Geometry: final body of the model. Coordinates: model frame, mm. Face numbers are marked on the shaded views. A direction names the side the tool comes from. Coordinates: 2 decimals unless noted, no trailing zeros. Loops run counter-clockwise (first coordinate to the right, second up) from the corner with the lowest first, then second, coordinate; pieces in that order, holes last. Notation, with made-up numbers: (28, 9.25) - (53, 9.25) arc R20 cw to (53, 45.25) - close; hole circle Ø5 at (47.5, -16.5). An arc over 180 degrees is marked (long way). Answer in a Markdown table with one row per item.
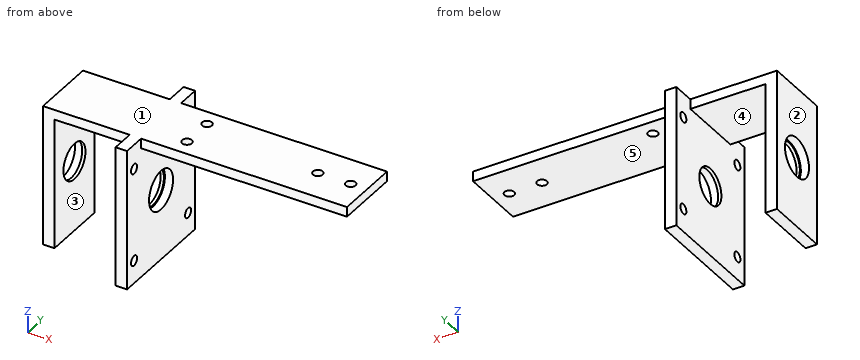
from build123d import *

# Parameters (mm, degrees)
SKETCH_1_W          = 20
SKETCH_1_H          = 20
SKETCH_1_R          = 1.5
SKETCH_1_W_2        = 23
SKETCH_1_W_3        = 3.5
EXTRUDE_1_DEPTH     = 3
EXTRUDE_2_DEPTH     = 40
SKETCH_2_R          = 1.5
CUT_EXTRUDE_1_DEPTH = 10
SKETCH_1_4_W        = 3.5
SKETCH_1_4_H        = 20
EXTRUDE_3_DEPTH     = 40
SKETCH_3_R          = 6
CUT_EXTRUDE_2_DEPTH = 38
SKETCH_4_R          = 6
SKETCH_4_R_2        = 5.5
EXTRUDE_4_DEPTH     = 1
SKETCH_5_R          = 6
SKETCH_5_R_2        = 5.5
EXTRUDE_5_DEPTH     = 1
SKETCH_7_R          = 1.5
CUT_EXTRUDE_4_DEPTH = 5


with BuildPart() as part:
    # Sketch 1 → Extrude 1 (new body)
    with BuildSketch(Plane.XY):
        Polygon((-10, -10.145751311), (-10, 9.854248689), (-53, 9.854248689), (-53, -0.145751311), (-53, -10.145751311), align=None)
        with Locations((0, -0.145751311)):
            Rectangle(SKETCH_1_W, SKETCH_1_H)
        with Locations((-5, -0.145751311)):
            Circle(SKETCH_1_R, mode=Mode.SUBTRACT)
        with Locations((5, -0.145751311)):
            Circle(SKETCH_1_R, mode=Mode.SUBTRACT)
        Polygon((-53, -0.145751311), (-53, 9.854248689), (-53, 16.854248689), (-56.5, 16.854248689), (-56.5, 9.854248689), (-56.5, -10.145751311), (-56.5, -17.145751311), (-53, -17.145751311), (-53, -10.145751311), align=None)
        with Locations((-68, -0.145751311)):
            Rectangle(SKETCH_1_W_2, SKETCH_1_H)
        with Locations((-81.25, -0.145751311)):
            Rectangle(SKETCH_1_W_3, SKETCH_1_H)
    extrude(amount=EXTRUDE_1_DEPTH)

    # Sketch 1_3 → Extrude 2 (add)
    with BuildSketch(Plane.XY):
        Polygon((-56.5, 16.854248689), (-56.5, 9.854248689), (-56.5, -10.145751311), (-56.5, -17.145751311), (-53, -17.145751311), (-53, -0.145751311), (-53, 16.854248689), align=None)
    extrude(amount=-EXTRUDE_2_DEPTH)

    # Sketch 2 → Cut-Extrude 1 (cut, symmetric)
    with BuildSketch(Plane(origin=(-53, 0, 0), x_dir=(0, 0, -1), z_dir=(-1, 0, 0))):
        with Locations((33, -13.354248689)):
            Circle(SKETCH_2_R)
        with Locations((4.5, 13.645751311)):
            Circle(SKETCH_2_R)
        with Locations((33, 13.645751311)):
            Circle(SKETCH_2_R)
        with Locations((4.5, -13.354248689)):
            Circle(SKETCH_2_R)
    extrude(amount=CUT_EXTRUDE_1_DEPTH, both=True, mode=Mode.SUBTRACT)

    # Sketch 1_4 → Extrude 3 (add)
    with BuildSketch(Plane.XY):
        with Locations((-81.25, -0.145751311)):
            Rectangle(SKETCH_1_4_W, SKETCH_1_4_H)
    extrude(amount=-EXTRUDE_3_DEPTH)

    # Sketch 3 → Cut-Extrude 2 (cut)
    with BuildSketch(Plane.ZY.offset(83)):
        with Locations((-18.5, -0.145751311)):
            Circle(SKETCH_3_R)
    extrude(amount=-CUT_EXTRUDE_2_DEPTH, mode=Mode.SUBTRACT)

    # Sketch 4 → Extrude 4 (add)
    with BuildSketch(Plane.ZY.offset(56.5)):
        with Locations((-18.5, -0.145751311)):
            Circle(SKETCH_4_R)
        with Locations((-18.5, -0.145751311)):
            Circle(SKETCH_4_R_2, mode=Mode.SUBTRACT)
    extrude(amount=-EXTRUDE_4_DEPTH)

    # Sketch 5 → Extrude 5 (add)
    with BuildSketch(Plane(origin=(-79.5, 0, 0), x_dir=(0, 0, -1), z_dir=(1, 0, 0))):
        with Locations((18.5, -0.145751311)):
            Circle(SKETCH_5_R)
        with Locations((18.5, -0.145751311)):
            Circle(SKETCH_5_R_2, mode=Mode.SUBTRACT)
    extrude(amount=-EXTRUDE_5_DEPTH)

    # Sketch 7 → Cut-Extrude 4 (cut)
    with BuildSketch(Plane.XY.offset(3)):
        with Locations((-42, 4.853948946)):
            Circle(SKETCH_7_R)
        with Locations((-42, -5.146051054)):
            Circle(SKETCH_7_R)
    extrude(amount=-CUT_EXTRUDE_4_DEPTH, mode=Mode.SUBTRACT)


solid = part.part
(1) Cut plane A-A on z = -33. Output: boundary loops of the cut face in (x, y).
Verdict:
| item | result |
|---|---|
| outline | (-83, -10.15) - (-79.5, -10.15) - (-79.5, 9.85) - (-83, 9.85) - close; (-56.5, -17.15) - (-53, -17.15) - (-53, -15.15) - (-56.5, -15.15) - close; (-56.5, -12.15) - (-53, -12.15) - (-53, 11.85) - (-56.5, 11.85) - close; (-56.5, 14.85) - (-53, 14.85) - (-53, 16.85) - (-56.5, 16.85) - close |
(2) Access query for the marked faces 4 and 5. Directions: +Z, -Z, +X, -X, +Y, -Y. A direction counts if a zero-diameter tool reaches every point of the face in a straight line with its end or side. Return the directions, or none.
Verdict:
| item | result |
|---|---|
| face 4 | -Z, +Y, -Y |
| face 5 | -Z, +X, +Y, -Y |
(3) Cut plane B-B on x = -5. Output: boundary loops of the cut face in (y, z), then the cut area to 3 significant figures.
Verdict:
| item | result |
|---|---|
| outline | (-10.15, 0) - (-1.65, 0) - (-1.65, 3) - (-10.15, 3) - close; (1.35, 0) - (9.85, 0) - (9.85, 3) - (1.35, 3) - close |
| area | 51.0 mm² |
(4) Pull-direction query (X, two-part tool) for the marked faces 1, 2 and 3; classes: pulls with the +X half, pulls with the -X half, needs draft (parallel to the pull), parting line crosses it, or undercut.
Verdict:
| item | result |
|---|---|
| face 1 | needs draft |
| face 2 | pulls with the -X half |
| face 3 | undercut |
(5) First-contact query: pin 1 Ø3 at (x, y) = (-62.5, 12) entering from -Z; pin 2 Ø14.5 at (y, z) = (-0.15, -18.5) entering from +X; pin 3 Ø16 at (x, y) = (-71, -3.5) entering from -Z; pin 4 Ø4 at (y, z) = (12.5, -6.5) entering from -X. Flat tips, straight axial feed; report the tip coordinate or a pass-through.
Verdict:
| item | result |
|---|---|
| pin 1 | passes through |
| pin 2 | stops at x = -53 |
| pin 3 | stops at z = 0 |
| pin 4 | stops at x = -56.5 |
(6) Cut plane C-C on z = -18.5. Output: boundary loops of the cut face in (x, y), then the cut area to 3 significant figures.
Verdict:
| item | result |
|---|---|
| outline | (-83, -10.15) - (-79.5, -10.15) - (-79.5, -5.65) - (-80.5, -5.65) - (-80.5, -6.15) - (-83, -6.15) - close; (-83, 5.85) - (-80.5, 5.85) - (-80.5, 5.35) - (-79.5, 5.35) - (-79.5, 9.85) - (-83, 9.85) - close; (-56.5, -17.15) - (-53, -17.15) - (-53, -6.15) - (-55.5, -6.15) - (-55.5, -5.65) - (-56.5, -5.65) - close; (-56.5, 5.35) - (-55.5, 5.35) - (-55.5, 5.85) - (-53, 5.85) - (-53, 16.85) - (-56.5, 16.85) - close |
| area | 107 mm² |
(7) Cut plane D-D on x = -45.5. Output: boundary loops of the cut face in (y, z), then the cut area to 3 significant figures.
Verdict:
| item | result |
|---|---|
| outline | (-10.15, 0) - (9.85, 0) - (9.85, 3) - (-10.15, 3) - close |
| area | 60.0 mm² |
(8) Ray query, probe 1 along Y at (x, z) = (-42, 1); probe 2 along Y at (x, z) = (-53.95, -4.5); probe 3 along X at (y, z) = (-2.5, -33). Return the intervals inside material, ascending.
Verdict:
| item | result |
|---|---|
| probe 1 | y = -10.15 to -6.65, -3.65 to 3.35, 6.35 to 9.85 |
| probe 2 | y = -17.15 to -15.15, -12.15 to 11.85, 14.85 to 16.85 |
| probe 3 | x = -83 to -79.5, -56.5 to -53 |
